```python
from build123d import *

# Parameters (mm, degrees)
BOSS_EXTRU_1_DEPTH     = 2
D_GAGEMENT_M3_51_D     = 3
D_GAGEMENT_M3_51_DEPTH = 2


with BuildPart() as part:
    # Esquisse1 → Boss.-Extru.1 (new body)
    with BuildSketch(Plane.XY):
        Polygon((27.15, 17.5), (34.85, 17.5), (34.85, -1.6), (27.15, -1.6), (27.15, -21.6), (-27.15, -21.6), (-27.15, 21.6), (27.15, 21.6), align=None)
    extrude(amount=BOSS_EXTRU_1_DEPTH)

    # Dégagement M3.51
    with Locations(Plane.XY.offset(2)):
        with Locations((-23.85, 18), (-23.85, -17.9), (-23.85, -17.8), (23.45, -17.9)):
            Hole(D_GAGEMENT_M3_51_D / 2, depth=D_GAGEMENT_M3_51_DEPTH)


solid = part.part
```
Could you check a few things on this model? Use its own coordinates, in mm. A direction names the side the tool comes from. Round coordinates to 2 decimals unless told otherwise and drop trailing zeros. Loops run counter-clockwise (first coordinate to the right, second up) from the corner with the lowest first, then second, coordinate; pieces in that order, holes last. Notation, with made-up numbers: M 60.5,61 L 84.5,61 A28 cw 84.5,96 Z; hole C 1,32.5 d2. An arc over 180 degrees is marked long. Put each result on its own line as item: value.
Q1. I need wall thicknesses on probe 1 along Y at (x, z) = (-23.85, 1.3); probe 2 along Y at (x, z) = (23.45, 1.1); probe 3 along Y at (x, z) = (30, 1.15). Which ranges of each line are inside material? Lowest first, please.
Check result:
probe 1: -21.6 to -19.4, -16.3 to 16.5, 19.5 to 21.6
probe 2: -21.6 to -19.4, -16.4 to 21.6
probe 3: -1.6 to 17.5
Q2. Imagine slicing it at A-A (x = -23.85). Write out the boundary of the cut face in (y, z), then the cut area to 3 significant figures.
Check result:
outline: M -21.6,0 L -19.4,0 L -19.4,2 L -21.6,2 Z; M -16.3,0 L 16.5,0 L 16.5,2 L -16.3,2 Z; M 19.5,0 L 21.6,0 L 21.6,2 L 19.5,2 Z
area: 74.2 mm2
Q3. Imagine slicing it at C-C (z = 1.1). Write out the boundary of the cut face in (x, y), then the cut area to 3 significant figures.
Check result:
outline: M -27.15,-21.6 L 27.15,-21.6 L 27.15,-1.6 L 34.85,-1.6 L 34.85,17.5 L 27.15,17.5 L 27.15,21.6 L -27.15,21.6 Z; hole M -25.35,-17.85 A1.5 ccw long -22.35,-17.85 A1.5 ccw long Z; hole C -23.85,18 d3; hole C 23.45,-17.9 d3
area: 2,470 mm2
Q4. For pin 1 (1 mm diameter, centred on y = 19, z = 1.5, fed in from +X); pin 2 (1 mm diameter, centred on x = 30.5, z = 1, fed in from +Y); pin 3 (0.6 mm diameter, centred on x = 29, z = 1, fed in from -Y), each with a flat end and sliding along its axis, tell me the tip position at first contact or that it passes through.
Check result:
pin 1: x = 27.15
pin 2: y = 17.5
pin 3: y = -1.6
Q5. On a 3-axis mill with a long thin cutter (end or side, diameter ignored), from which of +Z, -Z, +X, -X, +Y, -Y can I reach the whole of each face in a straight line? I mean faces 4 (the face through (34.85, 8, 1)), 5 (the face through (27.15, 20, 1)), 6 (the face through (0, 21.6, 1)), 7 (the face through (-23.8, -19.4, 1)), 8 (the face through (31, -1.6, 1)). Say none if no direction works.
Check result:
face 4: +Z, -Z, +X, +Y, -Y
face 5: +Z, -Z, +X, +Y
face 6: +Z, -Z, +X, -X, +Y
face 7: +Z, -Z
face 8: +Z, -Z, +X, -Y
Q6. Thinking about a two-plate mould opening in Y: for faces 1 (the face through (31, 17.5, 1)), 2 (the face through (4, 0, 0)), 3 (the face through (23.645, -16.413, 0.986)), which applies, released by +Y, released by -Y, zero draft, split by the parting line, or undercut?
Check result:
face 1: released by +Y
face 2: zero draft
face 3: undercut
Q7. Imagine slicing it at B-B (x = 23.45). Write out the boundary of the cut face in (y, z).
Check result:
outline: M -21.6,0 L -19.4,0 L -19.4,2 L -21.6,2 Z; M -16.4,0 L 21.6,0 L 21.6,2 L -16.4,2 Z
